Verification items for this drawing (mm, ordinates from the low corner). A direction names the side the tool comes from. Give positions to 0.01 mm unless a question says otherwise; leave off trailing zeros. Order: outer loops, then holes, each group sorted by start corner. A loop starts at its lowest first (then second) coordinate and runs counter-clockwise, first axis right, second up. Notation, with made-up numbers: M -2.75,-17.75 L 5.25,-17.75 A35 ccw 5.25,21.25 Z; hole C -6.75,-17 d8. An arc over 180 degrees is marked long. One line per question, with ' | ' between items. Start each with the question number.
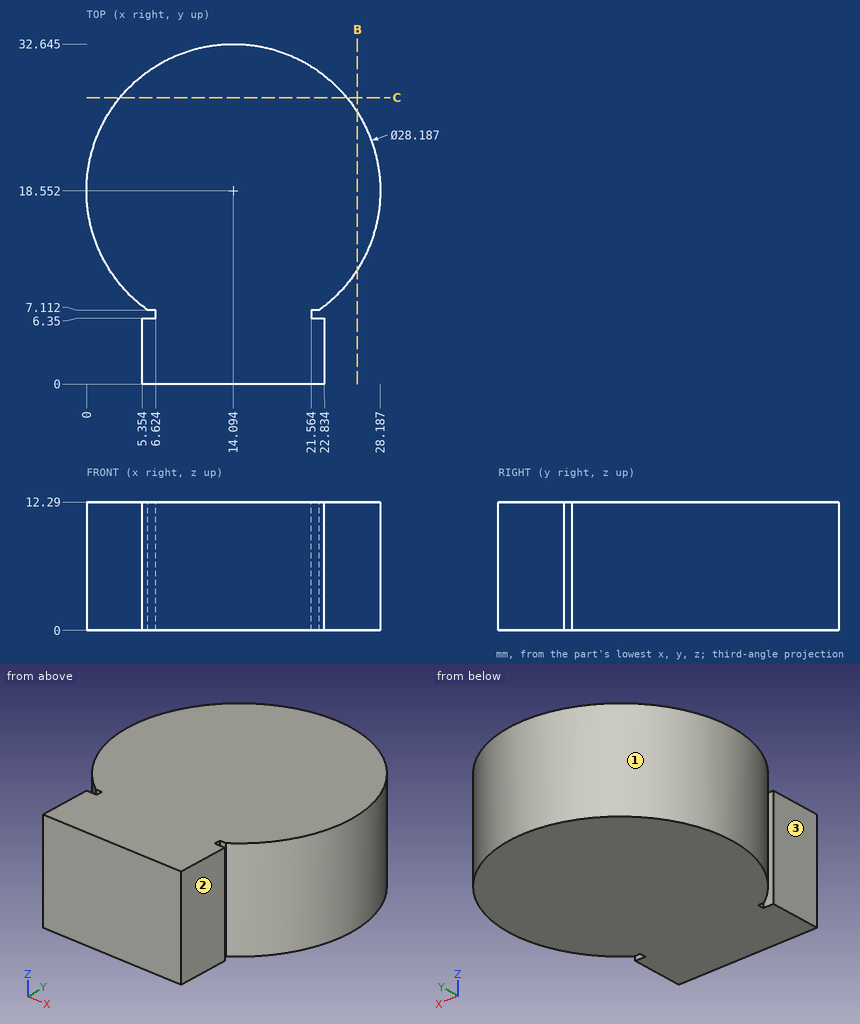
Item 1: Depth check by flat-ended pin: pin 1 (5 mm diameter, centred on y = 4, z = 10, fed in from -X); pin 2 (0.8 mm diameter, centred on y = 6.5, z = 4, fed in from +X); pin 3 (1.5 mm diameter, centred on y = 10, z = 4, fed in from -X). Enter the tip coordinate at first touch or a pass-through.
Item 2: Set-up check for the marked faces 1, 2 and 3: record each of +Z, -Z, +X, -X, +Y, -Y from which the full face is reachable in a straight line by a thin tool's end or side.
Item 3: Material ranges on line 1 along X through (y, z) = (4.5, 5); line 2 along Y through (x, z) = (14.5, 11.25); line 3 along Y through (x, z) = (3.5, 9.25) (1 decimal), recorded low to high.
Item 4: Cross-section at C-C, the plane y = 27.5. Record the cut outline in (x, z) (1 decimal).
Item 5: Cross-section at B-B, the plane x = 26. Record the cut outline in (y, z).
Outcome:
1) pin 1: stops at x = 5.35 | pin 2: stops at x = 22.83 | pin 3: stops at x = 2.36
2) face 1: +Z, -Z | face 2: +Z, -Z, +X, -Y | face 3: +Z, -Z, -X, -Y
3) line 1: x = 5.35 to 22.83 | line 2: y = 0 to 32.64 | line 3: y = 9.3 to 27.8
4) outline: M 3.2,0 L 25,0 L 25,12.3 L 3.2,12.3 Z
5) outline: M 11.01,0 L 26.09,0 L 26.09,12.29 L 11.01,12.29 Z
